```python
from build123d import *

# Parameters (mm, degrees)
BOSS_EXTRUDE1_DEPTH = 5
SKETCH3_W           = 2.5
SKETCH3_H           = 1.5
CUT_EXTRUDE1_DEPTH  = 172.058469536


with BuildPart() as part:
    # Sketch2 → Boss-Extrude1 (new body)
    with BuildSketch(Plane.XY.offset(-2.5)):
        Polygon((-70, -139.5), (-70, -131.5), (-40, -131.5), (-40, -134.5), (-55, -134.5), (-55, -139.5), (0, -139.5), (0, -150), (-10, -150), (-10, -153), (-5, -153), (-5, -156), (-15, -156), (-65, -144.5), (-70, -144.5), align=None)
    extrude(amount=-BOSS_EXTRUDE1_DEPTH)

    # Sketch3 → Cut-Extrude1 (cut, through all)
    with BuildSketch(Plane(origin=(0, 0, -7.5), x_dir=(-1, 0, 0), z_dir=(0, 0, -1))):
        with Locations((3.75, -140.25)):
            Rectangle(SKETCH3_W, SKETCH3_H)
    extrude(amount=-CUT_EXTRUDE1_DEPTH, mode=Mode.SUBTRACT)


solid = part.part
```
Can you work these out from the model? Positions are in its coordinate system, mm. A direction names the side the tool comes from. Give positions to 0.01 mm unless a question says otherwise; leave off trailing zeros. Write each loop counter-clockwise with the first axis right and the second up, starting at its lowest first coordinate (ties: lowest second). Pieces come first, ordered by that corner, then holes. Notation, with made-up numbers: (-20, 0.5) - (-12, 0.5) arc R30 cw to (-12, 38.5) - close; hole circle Ø4 at (30, 10). An arc over 180 degrees is marked (long way). Write item = value, one per line. Start each with the question number.
1. Thinking about a two-plate mould opening in X: for faces 1 (the face through (-5, -140, -5)), 2 (the face through (-10, -151, -5)), 3 (the face through (-35, -144, -2.5)), which applies, released by +X, released by -X, zero draft, split by the parting line, or undercut?
2. Please list where these lines run through material, in increasing order: line 1 (X direction, y = -136, z = -2.75); line 2 (Y direction, x = -11, z = -7.1); line 3 (X direction, y = -140.75, z = -3.1).
3. For pin 1 (3 mm diameter, centred on x = -41, z = -5.5, fed in from -Y) (3 decimals); pin 2 (1.6 mm diameter, centred on y = -140.5, z = -5, fed in from +X); pin 3 (2.5 mm diameter, centred on y = -138, z = -5, fed in from +X); pin 4 (2 mm diameter, centred on x = -23, z = -5.5, fed in from +Y), each with a flat end and sliding along its axis, tell me the tip position at first contact or that it passes through.
4. Imagine slicing it at A-A (x = -42). Please give me the cut outline in (y, z).
5. On a 3-axis mill with a long thin cutter (end or side, diameter ignored), from which of +Z, -Z, +X, -X, +Y, -Y can I reach the whole of each face in a straight line? I mean faces 4 (the face through (-5, -150, -5)), 5 (the face through (-40, -133, -5)), 6 (the face through (-5, -154, -5)), 7 (the face through (-4, -141, -5)). Say none if no direction works.
6. Imagine slicing it at D-D (x = -33). Please give me the cut outline in (y, z).
7. Imagine slicing it at C-C (y = -135.75). Please give me the cut outline in (x, z), and give its area (3 significant figures).
8. Imagine slicing it at B-B (z = -3.25). Please give me the cut outline in (x, y).
Worked answers:
q1.face_1 = undercut
q1.face_2 = released by +X
q1.face_3 = zero draft
q2.line_1 = -70 to -55
q2.line_2 = -156 to -139.5
q2.line_3 = -70 to -5, -2.5 to 0
q3.pin_1 = -150.365
q3.pin_2 = 0
q3.pin_3 = -55
q3.pin_4 = -139.5
q4.outline = (-149.79, -7.5) - (-139.5, -7.5) - (-139.5, -2.5) - (-149.79, -2.5) - close; (-134.5, -7.5) - (-131.5, -7.5) - (-131.5, -2.5) - (-134.5, -2.5) - close
q5.face_4 = +Z, -Z, +X
q5.face_5 = +Z, -Z, +X, +Y
q5.face_6 = +Z, -Z, +X, -Y
q5.face_7 = +Z, -Z, +Y
q6.outline = (-151.86, -7.5) - (-139.5, -7.5) - (-139.5, -2.5) - (-151.86, -2.5) - close
q7.outline = (-70, -7.5) - (-55, -7.5) - (-55, -2.5) - (-70, -2.5) - close
q7.area = 75.0 mm2
q8.outline = (-70, -144.5) - (-65, -144.5) - (-15, -156) - (-5, -156) - (-5, -153) - (-10, -153) - (-10, -150) - (0, -150) - (0, -139.5) - (-2.5, -139.5) - (-2.5, -141) - (-5, -141) - (-5, -139.5) - (-55, -139.5) - (-55, -134.5) - (-40, -134.5) - (-40, -131.5) - (-70, -131.5) - close
